```python
from build123d import *

# Parameters (mm, degrees)
F1_DEPTH      = 3
F2_W          = 4
F2_H          = 6.1803398875
F3_DEPTH      = 1
F5_DEPTH      = 8.0911699437
F5_DEPTH_BACK = 10.001
F6_T1_DEPTH   = 16.9244695544
F7_DEPTH      = 1
F8_R          = 5
F9_R          = 1


# Not quite as in the source:
# - a fillet or chamfer that OpenCascade refuses, or shapes differently, is made with other operations: its cross-section is extruded or revolved along the edge and cut away or added


with BuildPart() as f1:
    # F0 (on Top) → F1 (new body)
    with BuildSketch(Plane.XY):
        with BuildLine():
            ThreePointArc((10, 0), (7.5, 7.5), (0, 5))
            ThreePointArc((0, 5), (-7.5, 7.5), (-10, 0))
            Line((-10, 0), (0, -10))
            Line((0, -10), (10, 0))
        make_face()
    extrude(amount=F1_DEPTH)

    # F2 (on face) → F3 (join)
    with BuildSketch(Plane.XY.offset(3)):
        with BuildLine():
            ThreePointArc((0, 5), (-7.5, 7.5), (-10, 0))
            Line((-10, 0), (0, -10))
            Line((0, -10), (10, 0))
            ThreePointArc((10, 0), (7.5, 7.5), (0, 5))
        make_face()
        Rectangle(F2_W, F2_H, mode=Mode.SUBTRACT)
        Rectangle(F2_W, F2_H)
    extrude(amount=F3_DEPTH)

    # F4 (on Front) → F5 (cut, two sides)
    with BuildSketch(Plane.XZ) as f5_sk:
        with BuildLine():
            Line((0.75, 4), (-0.75, 4))
            Line((-0.75, 4), (-0.75, 3.7348469228))
            ThreePointArc((-0.75, 3.7348469228), (0, 1.95), (0.75, 3.7348469228))
            Line((0.75, 3.7348469228), (0.75, 4))
        make_face()
    extrude(amount=-F5_DEPTH, mode=Mode.SUBTRACT)
    extrude(f5_sk.sketch, amount=F5_DEPTH_BACK, mode=Mode.SUBTRACT)

    # F6: chamfer of 0.3 on 2 edges, made by hand

    # F6_s2 → F6_t1 (cut)
    with BuildSketch(Plane.XZ.offset(-6.902964658)):
        Polygon((1.05, 4), (0.75, 3.7), (0.75, 4), align=None)
        Polygon((-0.75, 3.7), (-1.05, 4), (-0.75, 4), align=None)
    extrude(amount=F6_T1_DEPTH, mode=Mode.SUBTRACT)

    # F7 (cut): a face of the model
    f7_faces = [f1.faces().sort_by_distance(p)[0] for p in [
        (0, 0.8210756438, 0),
    ]]
    extrude(f7_faces, amount=-F7_DEPTH, mode=Mode.SUBTRACT)

    # F8
    f8_edges = [f1.edges().sort_by_distance(p)[0] for p in [
        (10, 0, 2.5),
        (-10, 0, 2.5),
    ]]
    fillet(f8_edges, radius=F8_R)

    # F9
    f9_edges = [f1.edges().sort_by_distance(p)[0] for p in [
        (0, -10, 1.475),
    ]]
    fillet(f9_edges, radius=F9_R)


solid = f1.part
```
Can you work these out from the model? Positions are in its coordinate system, mm. Give positions to 0.01 mm unless a question says otherwise; leave off trailing zeros. Loops run counter-clockwise (first coordinate to the right, second up) from the corner with the lowest first, then second, coordinate; pieces in that order, holes last. Notation, with made-up numbers: M 4.5,34.25 L 17.5,34.25 A22 ccw 17.5,43.25 Z; hole C 62.5,44.25 d3. An arc over 180 degrees is marked long. One line per question, with ' | ' between items. Start each with the question number.
Q1. If we mould it in two halves opening along X, with no side actions, what happens to faces 1 (the flat face through (5, -5, 2)), 2 (the cylindrical face through (6, 8, 2)), 3 (the flat face through (-5, 2, 4))? For each: +X half, -X half, draft (parallel to the pull), parting line (faces both ways), or undercut.
Q2. If we section it at C-C (y = 7): Please give me the cut outline in (x, z), plus the area to 3 significant figures.
Q3. If we section it at B-B (y = -1.5): Please give me the cut outline in (x, z).
Q4. If I drill on line 1 (Z direction, x = 0, y = 1.25); line 2 (X direction, y = 5.25, z = 1.2); line 3 (X direction, y = -1, z = 3), over which ranges is the centre line in solid material (lowest first)? Write a range as from..to.
Q5. If we section it at A-A (z = 3): Please give me the cut outline in (x, y).
Q6. If we section it at D-D (x = -4): Please give me the cut outline in (y, z), plus the area to 3 significant figures.
Q7. For pin 1 Ø1 at (x, z) = (-7, 3.5) entering from -Y; pin 2 Ø1.3 at (x, z) = (0, 3) entering from +Y, each with a flat end and sliding along its axis, tell me the tip position at first contact or that it passes through.
Computed:
1) face 1: +X half | face 2: undercut | face 3: draft
2) outline: M -8.32,1 L -1.68,1 L -1.68,4 L -8.32,4 Z; M 1.68,1 L 8.32,1 L 8.32,4 L 1.68,4 Z | area: 39.8 mm²
3) outline: M -8.5,1 L 8.5,1 L 8.5,4 L 1.05,4 L 0.77,3.72 A1.05 cw long -0.77,3.72 L -1.05,4 L -8.5,4 Z
4) line 1: z = 1..1.95 | line 2: x = -9.87..-0.13, 0.13..9.87 | line 3: x = -9..-1.05, 1.05..9
5) outline: M -10.42,3.86 A5 ccw -9.11,-0.89 L -1.05,-8.95 L -1.05,6.46 A5.59 ccw Z; M 1.05,-8.95 L 9.11,-0.89 A5 ccw 10.42,3.86 A5.59 ccw 1.05,6.46 Z
6) outline: M -6,1 L 8,1 L 8,4 L -6,4 Z | area: 42.0 mm²
7) pin 1: stops at y = -3.5 | pin 2: passes through
